Geometry check sheet. Reference: the model listing, model coordinates, mm. Face numbers are marked on the shaded views. A direction names the side the tool comes from. Coordinates: 2 decimals unless noted, no trailing zeros. Order: outer loops, then holes, each group sorted by start corner. A loop starts at its lowest first (then second) coordinate and runs counter-clockwise, first axis right, second up. Notation, with made-up numbers: (3, 18.25) - (37, 18.25) arc R14 ccw to (37, 26.25) - close; hole circle Ø9 at (73.25, -16.75). An arc over 180 degrees is marked (long way). Return JSON: item names as keys, results as strings. Group by question number.
Item 1: Tool access check on the marked faces 1 and 2. Record the directions out of +Z, -Z, +X, -X, +Y, -Y that give a thin tool (end or side, any length) a straight path to the whole face; none if there is none.
Item 2: Section check D-D on x = 5.5. Enter the section's corners in (y, z).
Item 3: Section check A-A on z = -685.8. Enter the section's corners in (x, y).
Item 4: Section check B-B on y = 12.7. Enter the section's corners in (x, z), then the cut area to 3 significant figures.
Item 5: Scan lines: probe 1 along Z at (x, y) = (12.7, 1.25); probe 2 along Z at (x, y) = (1.75, 11); probe 3 along Y at (x, z) = (8.5, -699). Record each from-to range of solid material in increasing order.
Item 6: Gauge pin test, flat ends, axial feed: pin 1 (8 mm diameter, centred on x = 15.5, z = -679.5, fed in from +Y); pin 2 (6.5 mm diameter, centred on y = 12.7, z = -736.6, fed in from +X). Record the tip position at first contact, or that the pin passes through.
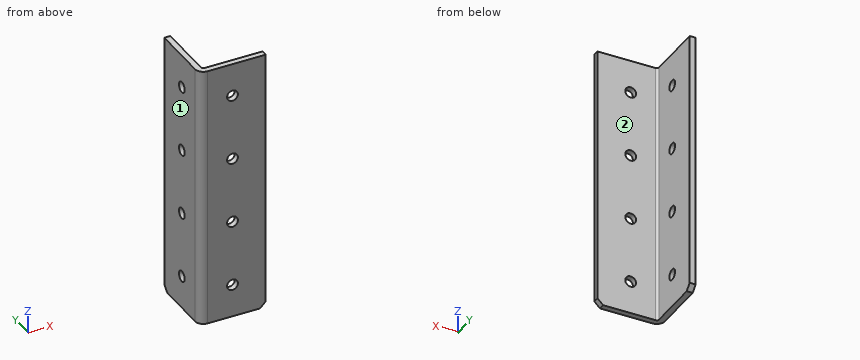
from build123d import *

# Parameters (mm, degrees)
SKETCH1_W                  = 25.4
SKETCH1_H                  = 1498.6
BOSS_EXTRUDE1_DEPTH        = 25.4
SKETCH2_W                  = 23.114
SKETCH2_H                  = 23.114
CUT_EXTRUDE1_DEPTH         = 1499.6
M3_5_CLEARANCE_HOLE1_D     = 4.1402
M3_5_CLEARANCE_HOLE1_DEPTH = 25.4
M3_5_CLEARANCE_HOLE2_D     = 4.1402
M3_5_CLEARANCE_HOLE2_DEPTH = 25.4
CHAMFER1_SIZE              = 2.159
FILLET1_R                  = 0.8128
FILLET2_R                  = 3.0988
SKETCH8_W                  = 95.882963774
SKETCH8_H                  = 79.338329604
CUT_EXTRUDE3_DEPTH         = 1397


with BuildPart() as part:
    # Sketch1 → Boss-Extrude1 (new body)
    with BuildSketch(Plane(origin=(0, 0, 0), x_dir=(0, -1, 0), z_dir=(-1, 0, 0))):
        with Locations((-12.7, 0)):
            Rectangle(SKETCH1_W, SKETCH1_H)
    extrude(amount=-BOSS_EXTRUDE1_DEPTH)

    # Sketch2 → Cut-Extrude1 (cut, through all)
    with BuildSketch(Plane(origin=(0, 0, -749.3), x_dir=(-1, 0, 0), z_dir=(0, 0, -1))):
        with Locations((-13.843, 13.843)):
            Rectangle(SKETCH2_W, SKETCH2_H)
    extrude(amount=-CUT_EXTRUDE1_DEPTH, mode=Mode.SUBTRACT)

    # M3.5 Clearance Hole1
    with Locations(Plane(origin=(0, 0, 0), x_dir=(-1, 0, 0), z_dir=(0, -1, 0))):
        with Locations((-12.7, 736.6), (-12.7, 711.2), (-12.7, 685.8), (-12.7, 660.4), (-12.7, 635), (-12.7, 609.6), (-12.7, 584.2), (-12.7, 558.8), (-12.7, 533.4), (-12.7, 508), (-12.7, 482.6), (-12.7, 457.2), (-12.7, 431.8), (-12.7, 406.4), (-12.7, 381), (-12.7, 355.6), (-12.7, 330.2), (-12.7, 304.8), (-12.7, 279.4), (-12.7, 254), (-12.7, 228.6), (-12.7, 203.2), (-12.7, 177.8), (-12.7, 152.4), (-12.7, 127), (-12.7, 101.6), (-12.7, 76.2), (-12.7, 50.8), (-12.7, 25.4), (-12.7, 0), (-12.7, -25.4), (-12.7, -50.8), (-12.7, -76.2), (-12.7, -101.6), (-12.7, -127), (-12.7, -152.4), (-12.7, -177.8), (-12.7, -203.2), (-12.7, -228.6), (-12.7, -254), (-12.7, -279.4), (-12.7, -304.8), (-12.7, -330.2), (-12.7, -355.6), (-12.7, -381), (-12.7, -406.4), (-12.7, -431.8), (-12.7, -457.2), (-12.7, -482.6), (-12.7, -508), (-12.7, -533.4), (-12.7, -558.8), (-12.7, -584.2), (-12.7, -609.6), (-12.7, -635), (-12.7, -660.4), (-12.7, -685.8), (-12.7, -711.2), (-12.7, -736.6)):
            Hole(M3_5_CLEARANCE_HOLE1_D / 2, depth=M3_5_CLEARANCE_HOLE1_DEPTH)

    # M3.5 Clearance Hole2
    with Locations(Plane.ZY):
        with Locations((711.2, 12.7), (736.6, 12.7), (685.8, 12.7), (660.4, 12.7), (635, 12.7), (609.6, 12.7), (584.2, 12.7), (558.8, 12.7), (533.4, 12.7), (508, 12.7), (482.6, 12.7), (457.2, 12.7), (431.8, 12.7), (406.4, 12.7), (381, 12.7), (355.6, 12.7), (330.2, 12.7), (304.8, 12.7), (279.4, 12.7), (254, 12.7), (228.6, 12.7), (203.2, 12.7), (177.8, 12.7), (152.4, 12.7), (127, 12.7), (101.6, 12.7), (76.2, 12.7), (50.8, 12.7), (25.4, 12.7), (0, 12.7), (-25.4, 12.7), (-50.8, 12.7), (-76.2, 12.7), (-101.6, 12.7), (-127, 12.7), (-152.4, 12.7), (-177.8, 12.7), (-203.2, 12.7), (-228.6, 12.7), (-254, 12.7), (-279.4, 12.7), (-304.8, 12.7), (-330.2, 12.7), (-355.6, 12.7), (-381, 12.7), (-406.4, 12.7), (-431.8, 12.7), (-457.2, 12.7), (-482.6, 12.7), (-508, 12.7), (-533.4, 12.7), (-558.8, 12.7), (-584.2, 12.7), (-609.6, 12.7), (-635, 12.7), (-660.4, 12.7), (-685.8, 12.7), (-711.2, 12.7), (-736.6, 12.7)):
            Hole(M3_5_CLEARANCE_HOLE2_D / 2, depth=M3_5_CLEARANCE_HOLE2_DEPTH)

    # Chamfer1
    chamfer1_edges = [part.edges().sort_by_distance(p)[0] for p in [
        (25.4, 1.143, -749.3),
        (1.143, 25.4, 749.3),
        (1.143, 25.4, -749.3),
        (25.4, 1.143, 749.3),
    ]]
    chamfer(chamfer1_edges, length=CHAMFER1_SIZE)

    # Fillet1
    fillet1_edges = [part.edges().sort_by_distance(p)[0] for p in [
        (2.286, 2.286, 0),
    ]]
    fillet(fillet1_edges, radius=FILLET1_R)

    # Fillet2
    fillet2_edges = [part.edges().sort_by_distance(p)[0] for p in [
        (0, 0, 0),
    ]]
    fillet(fillet2_edges, radius=FILLET2_R)

    # Sketch8 → Cut-Extrude3 (cut)
    with BuildSketch(Plane.XY.offset(749.3)):
        with Locations((2.286, 3.0988)):
            Rectangle(SKETCH8_W, SKETCH8_H)
    extrude(amount=-CUT_EXTRUDE3_DEPTH, mode=Mode.SUBTRACT)


solid = part.part
Computed:
{
 "1": {"face 1": "+Z, -Z, -X, +Y, -Y", "face 2": "+Z, -Z, +X, +Y"},
 "2": {"outline": "(0, -749.3) - (2.29, -749.3) - (2.29, -647.7) - (0, -647.7) - close"},
 "3": {"outline": "(0, 3.1) arc R3.1 ccw to (3.1, 0) - (10.63, 0) - (10.63, 2.29) - (3.1, 2.29) arc R0.81 cw to (2.29, 3.1) - (2.29, 10.63) - (0, 10.63) - close; (0, 14.77) - (2.29, 14.77) - (2.29, 25.4) - (0, 25.4) - close; (14.77, 0) - (25.4, 0) - (25.4, 2.29) - (14.77, 2.29) - close"},
 "4": {"outline": "(0, -749.3) - (2.29, -749.3) - (2.29, -738.67) - (0, -738.67) - close; (0, -734.53) - (2.29, -734.53) - (2.29, -713.27) - (0, -713.27) - close; (0, -709.13) - (2.29, -709.13) - (2.29, -687.87) - (0, -687.87) - close; (0, -683.73) - (2.29, -683.73) - (2.29, -662.47) - (0, -662.47) - close; (0, -658.33) - (2.29, -658.33) - (2.29, -647.7) - (0, -647.7) - close", "area": "194 mm²"},
 "5": {"probe 1": "z = -749.3 to -738.67, -734.53 to -713.27, -709.13 to -687.87, -683.73 to -662.47, -658.33 to -647.7", "probe 2": "z = -749.3 to -737.78, -735.42 to -712.38, -710.02 to -686.98, -684.62 to -661.58, -659.22 to -647.7", "probe 3": "y = 0 to 2.29"},
 "6": {"pin 1": "stops at y = 2.29", "pin 2": "stops at x = 2.29"}
}
